The figure shows three views and two pictorial views of one solid part (mm, origin at its lowest corner). Answer the questions. A direction names the side the tool comes from. Round coordinates to 2 decimals unless told otherwise and drop trailing zeros. Write each loop counter-clockwise with the first axis right and the second up, starting at its lowest first coordinate (ties: lowest second). Pieces come first, ordered by that corner, then holes. Notation, with made-up numbers: (4.25, 76) -> (9.25, 76) arc R16 ccw to (9.25, 85) -> close; hole circle Ø7 at (73, -16). An arc over 180 degrees is marked (long way). One line per item, written item: value.
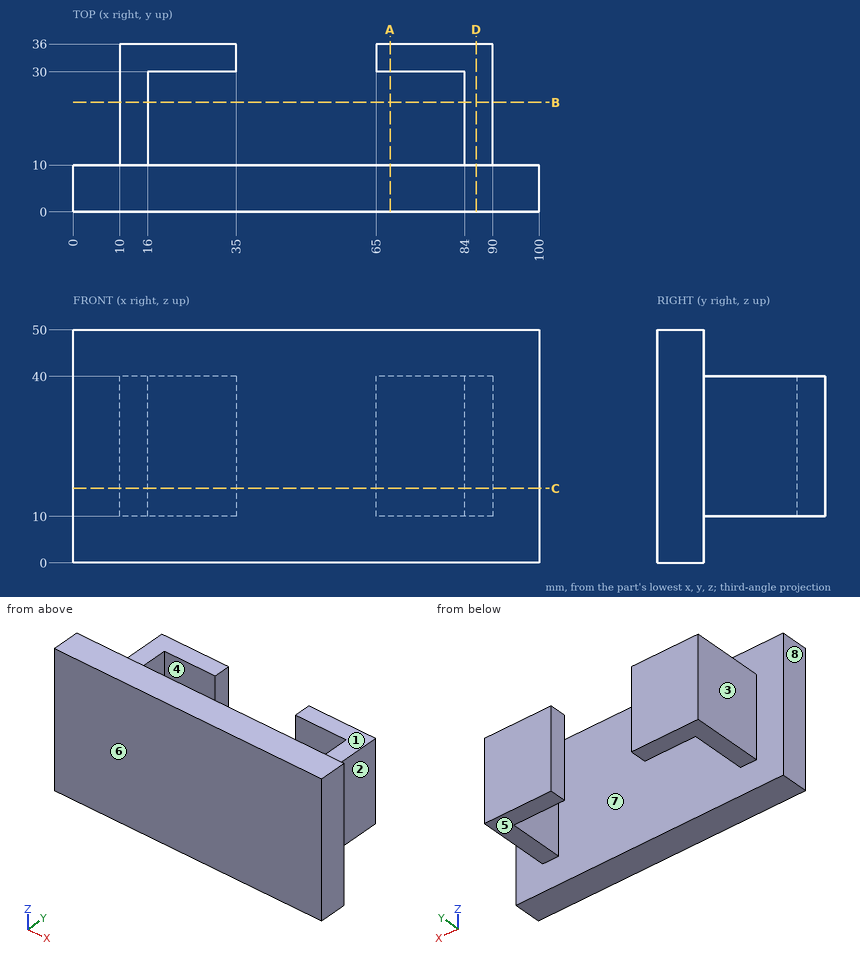
(1) Flat-ended cylindrical pins translate along their axes: pin 1 Ø9.5 at (x, z) = (26, 20.5) entering from -Y; pin 2 Ø20 at (x, y) = (81, 24) entering from +Z; pin 3 Ø6 at (y, z) = (18.5, 22) entering from -X; pin 4 Ø1.8 at (y, z) = (32.5, 22) entering from +X. Find the tip coordinate at first contact, or state that the pin passes through.
Reported:
pin 1: stops at y = 0
pin 2: stops at z = 40
pin 3: stops at x = 10
pin 4: stops at x = 90
(2) A tool of negligible diameter and unlimited length cuts with its end or side. For the marked faces 1, 2, 3, 4 and 5, from which of +Z, -Z, +X, -X, +Y, -Y can it reach the whole face along a straight path? Write none if from no direction.
Reported:
face 1: +Z, +X, -X, +Y
face 2: +Z, -Z, +X, +Y
face 3: +Z, -Z, -X, +Y
face 4: +Z, -Z
face 5: -Z, +X, -X, +Y
(3) For a pull along X with two mould halves and no side action, classify the marked faces 6, 7 and 8 as pulls with the +X half, pulls with the -X half, needs draft (parallel to the pull), parting line crosses it, or undercut.
Reported:
face 6: needs draft
face 7: undercut
face 8: pulls with the -X half
(4) Find section B-B on y = 23.5. Give the vertices of the cut face in (x, z).
Reported:
outline: (10, 10) -> (16, 10) -> (16, 40) -> (10, 40) -> close; (84, 10) -> (90, 10) -> (90, 40) -> (84, 40) -> close
(5) Find section A-A on x = 68. Give the vertices of the cut face in (y, z), plus the area to 3 significant figures.
Reported:
outline: (0, 0) -> (10, 0) -> (10, 50) -> (0, 50) -> close; (30, 10) -> (36, 10) -> (36, 40) -> (30, 40) -> close
area: 680 mm2
(6) Consider probe 1 along Y at (x, z) = (83, 13); probe 2 along X at (y, z) = (12, 25.5); probe 3 along X at (y, z) = (34.5, 12). Determine where each line is inside the solid, lowest interval first.
Reported:
probe 1: y = 0 to 10, 30 to 36
probe 2: x = 10 to 16, 84 to 90
probe 3: x = 10 to 35, 65 to 90
(7) Find section D-D on x = 86.5. Give the vertices of the cut face in (y, z).
Reported:
outline: (0, 0) -> (10, 0) -> (10, 10) -> (36, 10) -> (36, 40) -> (10, 40) -> (10, 50) -> (0, 50) -> close
(8) Find section C-C on z = 16. Give the vertices of the cut face in (x, y).
Reported:
outline: (0, 0) -> (100, 0) -> (100, 10) -> (90, 10) -> (90, 36) -> (65, 36) -> (65, 30) -> (84, 30) -> (84, 10) -> (16, 10) -> (16, 30) -> (35, 30) -> (35, 36) -> (10, 36) -> (10, 10) -> (0, 10) -> close
